Source: three-view drawing plus pictorial views. Frame: mm from the lowest corner of the part. Coordinates: 2 decimals unless noted, no trailing zeros. Order: outer loops, then holes, each group sorted by start corner. A loop starts at its lowest first (then second) coordinate and runs counter-clockwise, first axis right, second up. Notation, with made-up numbers: (25, 84.5) -> (68, 84.5) arc R32 ccw to (68, 114.5) -> close; hole circle Ø7 at (-40, 60.25). An arc over 180 degrees is marked (long way). One line per question, with ' | ' between items.
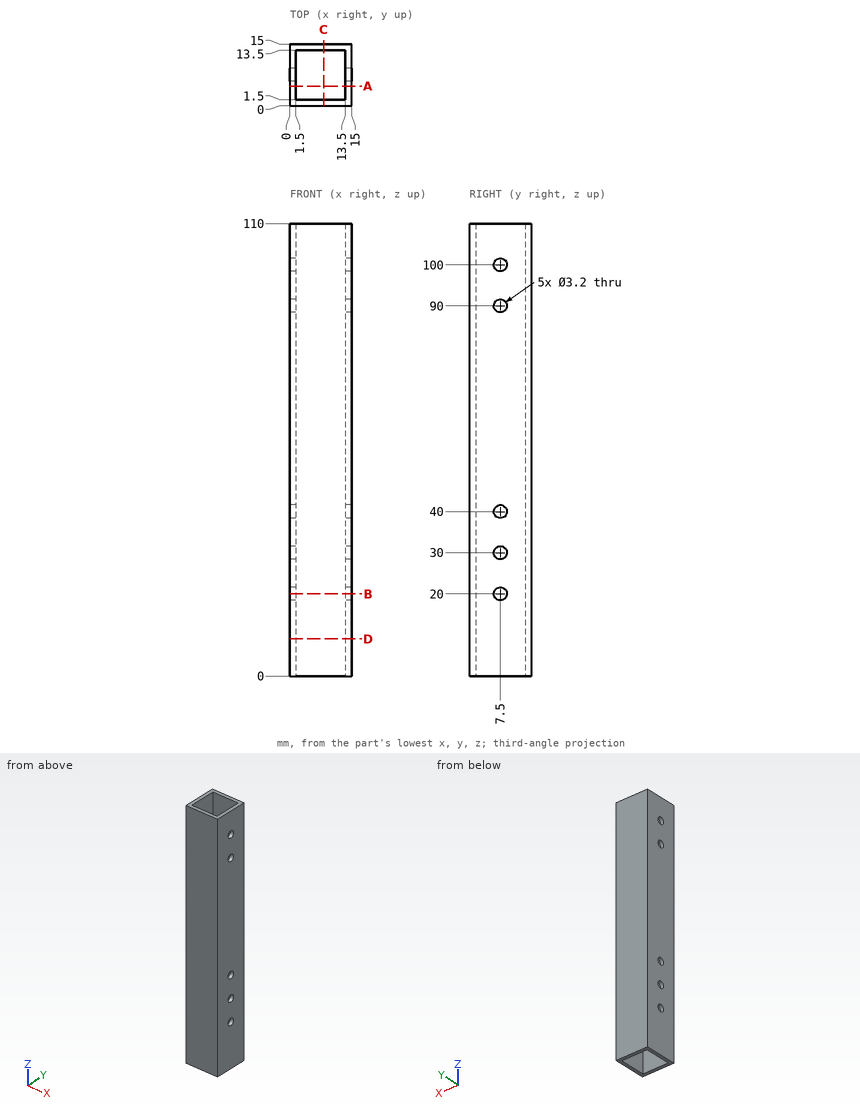
1. Ray query, line 1 (Z direction, x = 0.8, y = 7.5); line 2 (X direction, y = 5.5, z = 47.5). Return the intervals inside material, ascending. Write a range as [from, to].
Recorded:
line 1: z = [0, 18.4], [21.6, 28.4], [31.6, 38.4], [41.6, 88.4], [91.6, 98.4], [101.6, 110] | line 2: x = [0, 1.5], [13.5, 15]
2. Cut plane B-B, the plane z = 20. Return loops of the section in (x, y), and give its area (3 significant figures).
Recorded:
outline: (0, 0) -> (15, 0) -> (15, 5.9) -> (13.5, 5.9) -> (13.5, 1.5) -> (1.5, 1.5) -> (1.5, 5.9) -> (0, 5.9) -> close; (0, 9.1) -> (1.5, 9.1) -> (1.5, 13.5) -> (13.5, 13.5) -> (13.5, 9.1) -> (15, 9.1) -> (15, 15) -> (0, 15) -> close | area: 71.4 mm^2
3. Cut plane D-D, the plane z = 9. Return loops of the section in (x, y).
Recorded:
outline: (0, 0) -> (15, 0) -> (15, 15) -> (0, 15) -> close; hole (1.5, 1.5) -> (13.5, 1.5) -> (13.5, 13.5) -> (1.5, 13.5) -> close
4. Cut plane A-A, the plane y = 4.75. Return loops of the section in (x, z), and give its area (3 significant figures).
Recorded:
outline: (0, 0) -> (1.5, 0) -> (1.5, 110) -> (0, 110) -> close; (13.5, 0) -> (15, 0) -> (15, 110) -> (13.5, 110) -> close | area: 330 mm^2
5. Pin query (flat end, axial travel): pin 1 Ø1.9 at (y, z) = (7.5, 30) entering from -X. Return the tip coordinate at first contact, or that it passes through.
Recorded:
pin 1: passes through
